Part model, mm, in its own coordinate system. Face numbers are marked on the shaded views. Coordinates: 2 decimals unless noted, no trailing zeros. Order: outer loops, then holes, each group sorted by start corner. A loop starts at its lowest first (then second) coordinate and runs counter-clockwise, first axis right, second up. Notation, with made-up numbers: (14, 3.25) - (55, 3.25) arc R27 cw to (55, 20.25) - close; hole circle Ø8 at (25.5, -25.75). An arc over 180 degrees is marked (long way). Use a Markdown table: item, result. Add a question column.
1) Saw through at D-D on x = 1.15. List the corners of the cut face in (y, z).
2) Two-plate mould, pull along Y, no slides. Class the marked faces 1, 2 and 3: +Y half, -Y half, draft (parallel to the pull), parting line (faces both ways), or undercut.
3) Drop flat-ended pins along their axis: P1, Ø0.7, axis at x = 0, y = -1, coming from the +Z side; P2, Ø1.5, axis at x = 0, z = -4.5, coming from the +Y side; P3, Ø0.5, axis at x = 0, z = -4, coming from the -Y side. Give the stop position or say it passes through.
4) Saw through at B-B on z = 2.5. List the corners of the cut face in (x, y).
5) Wall check: L1, parallel to Z at x = -0.8, y = -1.3; L2, parallel to X at y = 0, z = 2.85. Give the ranges that are in metal, low to high. Write a range as [from, to].
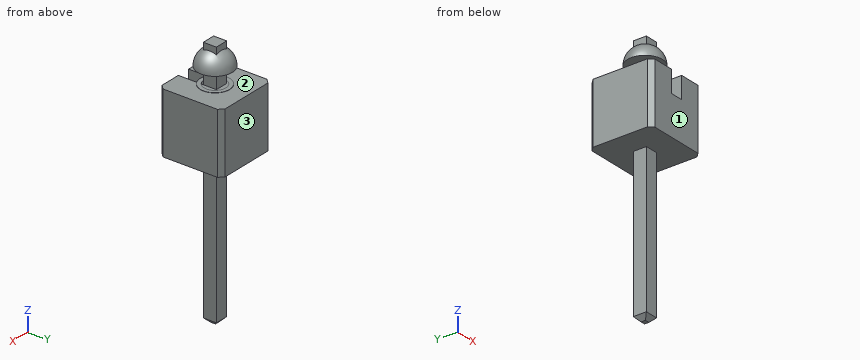
```python
from build123d import *

# Parameters (mm, degrees)
ESQUISSE1_W             = 0.6
ESQUISSE1_H             = 0.6
BOSS_EXTRU_1_DEPTH      = 2.8
ESQUISSE2_W             = 0.6
ESQUISSE2_H             = 1.15
ENL_V_MAT_EXTRU_1_DEPTH = 1
BOSS_EXTRU_2_DEPTH      = 0.75
BOSS_EXTRU_2_DEPTH_BACK = 9.8
ESQUISSE3_W             = 0.6
ESQUISSE3_H             = 0.6
CHANFREIN1_SIZE         = 0.2
ESQUISSE4_R             = 0.674645205
ESQUISSE4_R_2           = 0.5
BOSS_EXTRU_3_DEPTH      = 0.01
R_VOLUTION1_ANGLE       = 180
ESQUISSE6_W             = 0.6
ESQUISSE6_H             = 0.6
BOSS_EXTRU_4_DEPTH      = 1


with BuildPart() as part:
    # Esquisse1 → Boss.-Extru.1 (new body)
    with BuildSketch(Plane.XY):
        Polygon((-1.25, 1.45), (-1.45, 1.25), (-1.45, -1.25), (-1.25, -1.45), (1.25, -1.45), (1.45, -1.25), (1.45, 1.25), (1.25, 1.45), align=None)
        Rectangle(ESQUISSE1_W, ESQUISSE1_H, mode=Mode.SUBTRACT)
    extrude(amount=BOSS_EXTRU_1_DEPTH)

    # Esquisse2 → Enlèv. mat.-Extru.1 (cut)
    with BuildSketch(Plane.XY.offset(2.8)):
        with Locations((0, -0.875)):
            Rectangle(ESQUISSE2_W, ESQUISSE2_H)
    extrude(amount=-ENL_V_MAT_EXTRU_1_DEPTH, mode=Mode.SUBTRACT)

    # Esquisse3 → Boss.-Extru.2 (add, two sides: drawn at the far end of the back side and taken through both)
    with BuildSketch(Plane.XY.offset(2.8).offset(-BOSS_EXTRU_2_DEPTH_BACK)):
        Rectangle(ESQUISSE3_W, ESQUISSE3_H)
    extrude(amount=BOSS_EXTRU_2_DEPTH + BOSS_EXTRU_2_DEPTH_BACK)

    # Chanfrein1
    chanfrein1_edges = [part.edges().sort_by_distance(p)[0] for p in [
        (0, -0.3, -7),
        (0.3, 0, -7),
        (-0.3, 0, -7),
        (0, 0.3, -7),
    ]]
    chamfer(chanfrein1_edges, length=CHANFREIN1_SIZE)

    # Esquisse4 → Boss.-Extru.3 (add)
    with BuildSketch(Plane.XY.offset(2.8)):
        with Locations(Location((0, 0, 0), (0, 0, 243.597249523))):
            Circle(ESQUISSE4_R)
        with Locations(Location((0, 0, 0), (0, 0, 233.130102354))):
            Circle(ESQUISSE4_R_2, mode=Mode.SUBTRACT)
    extrude(amount=BOSS_EXTRU_3_DEPTH)

    # Esquisse5 → Révolution1 (revolve)
    with BuildSketch(Plane.XY.offset(3.55)):
        with BuildLine():
            Line((0.8, 0), (-0.8, 0))
            ThreePointArc((-0.8, 0), (0, 0.8), (0.8, 0))
        make_face()
    revolve(axis=Axis((0.8, 0, 3.55), (1, 0, 0)), revolution_arc=R_VOLUTION1_ANGLE)

    # Esquisse6 → Boss.-Extru.4 (add)
    with BuildSketch(Plane(origin=(0, 0, 3.55), x_dir=(-1, 0, 0), z_dir=(0, 0, -1))):
        Rectangle(ESQUISSE6_W, ESQUISSE6_H)
    extrude(amount=-BOSS_EXTRU_4_DEPTH)


solid = part.part
```
Results are:
| question | item | result |
|---|---|---|
| 1 | outline | (-1.45, 0) - (1.45, 0) - (1.45, 2.8) - (-1.45, 2.8) - close |
| 2 | face 1 | -Y half |
| 2 | face 2 | draft |
| 2 | face 3 | +Y half |
| 3 | P1 | z = 4.02 |
| 3 | P2 | y = 0.3 |
| 3 | P3 | y = -0.3 |
| 4 | outline | (-1.45, -1.25) - (-1.25, -1.45) - (-0.3, -1.45) - (-0.3, -0.3) - (0.3, -0.3) - (0.3, -1.45) - (1.25, -1.45) - (1.45, -1.25) - (1.45, 1.25) - (1.25, 1.45) - (-1.25, 1.45) - (-1.45, 1.25) - close |
| 5 | L1 | [0, 2.8] |
| 5 | L2 | [-0.3, 0.3] |
